Here's how the part is built. I have some questions about the finished solid (model axes, mm). Face numbers are marked on the shaded views. A direction names the side the tool comes from. Round coordinates to 2 decimals unless told otherwise and drop trailing zeros. Order: outer loops, then holes, each group sorted by start corner. A loop starts at its lowest first (then second) coordinate and runs counter-clockwise, first axis right, second up. Notation, with made-up numbers: (-14.75, 52.5) -> (26.25, 52.5) arc R8 ccw to (26.25, 61.5) -> close; hole circle Ø6 at (-35.5, 61). An arc over 180 degrees is marked (long way). Use a Markdown table: item, result. Add a question column.
(1) Thinking about a two-plate mould opening in X: for the marked faces 1, 2 and 3, which applies, pulls with the +X half, pulls with the -X half, needs draft (parallel to the pull), parting line crosses it, or undercut?
(2) I want a section at D-D, the plane y = 3. Please give me the cut outline in (x, z).
(3) I want a section at C-C, the plane z = 29.5. Please give me the cut outline in (x, y), then the cut area to 3 significant figures.
(4) If I drill on probe 1 along Y at (x, z) = (0, 43); probe 2 along X at (y, z) = (0, 19.5); probe 3 along X at (y, z) = (7, 14.5), over which ranges is the centre line in solid material (lowest first)?
(5) I'm going to push flat-ended pins straight in: P1, Ø4, axis at x = -26.5, z = 30, coming from the -Y side; P2, Ø5.5, axis at x = 45.5, z = 6, coming from the -Y side; P3, Ø11.5, axis at x = -4.5, y = 6.5, coming from the +Z side; P4, Ø15, axis at x = 0, y = 0, coming from the +Z side. Where does each tip first touch, or does it pass through?
(6) I want a section at B-B, the plane x = 65. Please give me the cut outline in (y, z) (3 decimals), then the cut area to 3 significant figures.
(7) On a 3-axis mill with a long thin cutter (end or side, diameter ignored), from which of +Z, -Z, +X, -X, +Y, -Y can I reach the whole of each face in a straight line? I mean the marked faces 4, 5, 6 and 7. Say none if no direction works.
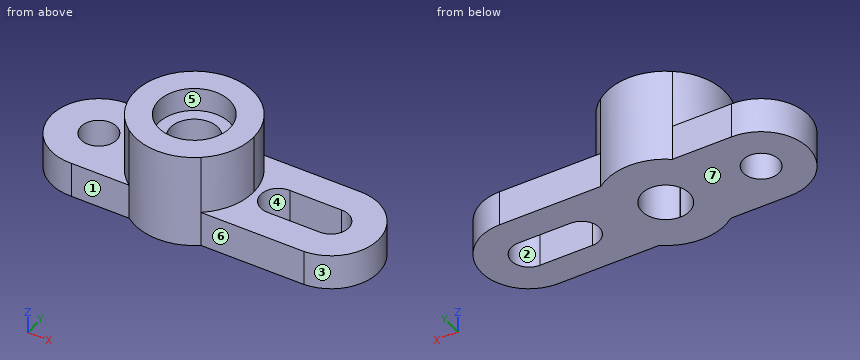
from build123d import *

# Parameters (mm, degrees)
F0_R     = 19.05
F1_DEPTH = 50.8
F2_DEPTH = 38.1
F0_R_2   = 9.525
F3_DEPTH = 19.05


with BuildPart() as f1:
    # F0 (on Top) → F1 (new body)
    with BuildSketch(Plane.XY):
        with BuildLine():
            ThreePointArc((19.075155, -25.381114), (28.405093, -14.184963), (31.75, 0))
            ThreePointArc((31.75, 0), (28.398153, 14.198852), (19.050322, 25.399759))
            ThreePointArc((19.050322, 25.399759), (-0.000142, 31.75), (-19.050549, 25.399588))
            ThreePointArc((-19.050549, 25.399588), (-31.749996, 0.015384), (-19.075155, -25.381114))
            ThreePointArc((-19.075155, -25.381114), (0, -31.75), (19.075155, -25.381114))
        make_face()
        Circle(F0_R, mode=Mode.SUBTRACT)
    extrude(amount=F1_DEPTH)

    # F0 (on Top) → F2 (join)
    with BuildSketch(Plane.XY):
        Circle(F0_R)
        with BuildLine():
            ThreePointArc((-0.198518, -12.698448), (0.00023, 12.7), (0.198058, -12.698456))
            Line((0.198058, -12.698456), (-0.198518, -12.698448))
        make_face(mode=Mode.SUBTRACT)
    extrude(amount=F2_DEPTH)

    # F0 (on Top) → F3 (join)
    with BuildSketch(Plane.XY):
        with BuildLine():
            ThreePointArc((19.050322, 25.399759), (28.398153, 14.198852), (31.75, 0))
            ThreePointArc((31.75, 0), (28.405093, -14.184963), (19.075155, -25.381114))
            Line((19.075155, -25.381114), (71.918698, -25.381114))
            Line((71.918698, -25.381114), (73.877302, -25.381114))
            ThreePointArc((73.877302, -25.381114), (98.293277, 0.489799), (72.897886, 25.4))
            Line((72.897886, 25.4), (19.050322, 25.399759))
        make_face()
        with BuildLine():
            ThreePointArc((44.831, -9.525), (35.306985, 0.136988), (45.104947, 9.52106))
            Line((45.104947, 9.52106), (72.497053, 9.52106))
            ThreePointArc((72.497053, 9.52106), (82.295015, 0.136988), (72.771, -9.525))
            Line((72.771, -9.525), (44.831, -9.525))
        make_face(mode=Mode.SUBTRACT)
        with BuildLine():
            ThreePointArc((-19.075155, -25.381114), (-31.749996, 0.015384), (-19.050549, 25.399588))
            Line((-19.050549, 25.399588), (-50.63229, 25.399446))
            ThreePointArc((-50.63229, 25.399446), (-76.196757, -0.4059), (-49.820698, -25.381114))
            Line((-49.820698, -25.381114), (-19.075155, -25.381114))
        make_face()
        with BuildLine():
            ThreePointArc((-50.54993, -12.697538), (-50.80023, -12.7), (-51.05053, -12.697529))
            Line((-51.05053, -12.697529), (-50.54993, -12.697538))
        make_face(mode=Mode.SUBTRACT)
        with Locations((-50.8, 0)):
            Circle(F0_R_2, mode=Mode.SUBTRACT)
    extrude(amount=F3_DEPTH)


solid = f1.part
Taken from the geometry:
| question | item | result |
|---|---|---|
| 1 | face 1 | needs draft |
| 1 | face 2 | undercut |
| 1 | face 3 | pulls with the +X half |
| 2 | outline | (-76.02, 0) -> (-59.84, 0) -> (-59.84, 19.05) -> (-76.02, 19.05) -> close; (-41.76, 0) -> (-12.34, 0) -> (-12.34, 38.1) -> (-18.81, 38.1) -> (-18.81, 50.8) -> (-31.61, 50.8) -> (-31.61, 19.05) -> (-41.76, 19.05) -> close; (12.34, 0) -> (35.79, 0) -> (35.79, 19.05) -> (31.61, 19.05) -> (31.61, 50.8) -> (18.81, 50.8) -> (18.81, 38.1) -> (12.34, 38.1) -> close; (81.81, 0) -> (98.12, 0) -> (98.12, 19.05) -> (81.81, 19.05) -> close |
| 3 | outline | (-19.08, -25.38) arc R31.75 ccw to (19.08, -25.38) arc R31.75 ccw to (31.75, 0) arc R31.75 ccw to (19.05, 25.4) arc R31.75 ccw to start; hole (-0.2, -12.7) -> (0.2, -12.7) arc R12.7 ccw (long way) to start |
| 3 | area | 2,660 mm2 |
| 4 | probe 1 | y = -31.75 to -19.05, 19.05 to 31.75 |
| 4 | probe 2 | x = -31.75 to -12.7, 12.7 to 31.75 |
| 4 | probe 3 | x = -75.22 to -57.26, -44.34 to -10.6, 10.6 to 38.37, 79.23 to 97.31 |
| 5 | P1 | stops at y = -20.19 |
| 5 | P2 | stops at y = -25.38 |
| 5 | P3 | stops at z = 38.1 |
| 5 | P4 | passes through |
| 6 | outline | (-25.381, 0) -> (-9.525, 0) -> (-9.525, 19.05) -> (-25.381, 19.05) -> close; (9.521, 0) -> (25.4, 0) -> (25.4, 19.05) -> (9.521, 19.05) -> close |
| 6 | area | 605 mm2 |
| 7 | face 4 | +Z, -Z |
| 7 | face 5 | +Z |
| 7 | face 6 | +Z, -Z, +X, -Y |
| 7 | face 7 | -Z, +X, -X, +Y, -Y |
